from build123d import *

# Parameters (mm, degrees)
CROQUIS1_R              = 2.1
SALIENTE_EXTRUIR1_DEPTH = 4
CROQUIS1_6_R            = 2.1
SALIENTE_EXTRUIR3_DEPTH = 12.65
REDONDEO1_R             = 10


with BuildPart() as part:
    # Croquis1 → Saliente-Extruir1 (new body)
    with BuildSketch(Plane.XY):
        with BuildLine():
            ThreePointArc((10, 54), (0, 64), (-10, 54))
            Line((-10, 54), (-10, -54))
            ThreePointArc((-10, -54), (0, -64), (10, -54))
            Line((10, -54), (10, 54))
        make_face()
        with Locations((0, 54)):
            Circle(CROQUIS1_R, mode=Mode.SUBTRACT)
        with BuildLine():
            Line((6, 38), (6, 22))
            Line((6, 22), (-6, 34))
            Line((-6, 34), (-6, 38))
            ThreePointArc((-6, 38), (0, 44), (6, 38))
        make_face(mode=Mode.SUBTRACT)
        Polygon((6, 16), (6, -16), (-6, -4), (-6, 4), align=None, mode=Mode.SUBTRACT)
        with BuildLine():
            Line((6, -22), (6, -38))
            ThreePointArc((6, -38), (0, -44), (-6, -38))
            Line((-6, -38), (-6, -34))
            Line((-6, -34), (6, -22))
        make_face(mode=Mode.SUBTRACT)
        Polygon((-6, -31), (-6, -7), (6, -19), align=None, mode=Mode.SUBTRACT)
        Polygon((-6, 7), (-6, 31), (6, 19), align=None, mode=Mode.SUBTRACT)
        with Locations((0, -54)):
            Circle(CROQUIS1_R, mode=Mode.SUBTRACT)
    extrude(amount=SALIENTE_EXTRUIR1_DEPTH)

    # Croquis1<6> → Saliente-Extruir3 (add)
    with BuildSketch(Plane.XY):
        with BuildLine():
            Line((10, 47.95), (10, 54))
            ThreePointArc((10, 54), (0, 64), (-10, 54))
            Line((-10, 54), (-10, 47.95))
            Line((-10, 47.95), (10, 47.95))
        make_face()
        with Locations((0, 54)):
            Circle(CROQUIS1_6_R, mode=Mode.SUBTRACT)
    extrude(amount=SALIENTE_EXTRUIR3_DEPTH)

    # Redondeo1
    # the kernel refuses this fillet: 10 mm, written as the material it adds along each edge
    with BuildSketch(Plane(origin=(10, 47.95, 4), x_dir=(0, 0, 1), z_dir=(-1, 0, 0))) as redondeo1_piece_1_section:
        with BuildLine():
            CenterArc((10, -9.908455985), REDONDEO1_R, 97.758619889, 82.241380111)
            Line((0, -9.908455985), (-0.2, -9.908455985))
            Line((-0.2, -9.908455985), (-0.2, 0))
            Line((-0.2, 0), (0, 0.2))
            ThreePointArc((0, 0.2), (4.325, 0.2), (8.623, 0.19816912))
            Line((8.623, 0.19816912), (8.65, 0))
        make_face()
    redondeo1_piece_1 = extrude(amount=20, mode=Mode.PRIVATE)
    redondeo1_piece_1 = redondeo1_piece_1 - Plane(origin=(0, 38, 6.259394391), x_dir=(-1, 0, 0), z_dir=(0, 0, -1)) * Cylinder(6, 80, mode=Mode.PRIVATE)
    add(redondeo1_piece_1)


solid = part.part
Model file for the job. Use its own axes, mm. A direction names the side the tool comes from. Coordinates: 2 decimals unless noted, no trailing zeros. Order: outer loops, then holes, each group sorted by start corner. A loop starts at its lowest first (then second) coordinate and runs counter-clockwise, first axis right, second up. Notation, with made-up numbers: (0, -37) -> (50, -37) arc R20 ccw to (50, -32) -> close; hole circle Ø11 at (50.5, 5.25). An arc over 180 degrees is marked (long way). Return JSON: item names as keys, results as strings. Group by question number.
Item 1: Saw through at D-D on z = 7.75. Write the cut outline in (x, y).
Item 2: Tool access for faces 1 (the flat face through (2, 56, 12.65)), 2 (the flat face through (6, 30, 2)), 3 (the flat face through (2, -24, 4)): list every direction of +Z, -Z, +X, -X, +Y, -Y with a clear straight run to the whole face (end or side of a thin tool).
Item 3: Saw through at C-C on z = 2.5. Write the cut outline in (x, y), then the cut area to 3 significant figures.
Item 4: Pull direction X, two halves, no side cores. Call faces 4 (the flat face through (10, 12.8, 3.6)), 5 (the flat face through (-6, -36, 2)), 6 (the cylindrical face through (0, -64, 2)), 7 (the flat face through (-7, 1, 0)): pulls with the +X half, pulls with the -X half, needs draft (parallel to the pull), parting line crosses it, or undercut.
Item 5: Saw through at B-B on x = 0. State how many separate pieces and enclosed holes the cut face has, then the cut area to 3 significant figures.
Item 6: Flat gauge pins, fed straight in: P1, Ø5, axis at x = -3, z = 9.5, coming from the -Y side; P2, Ø3, axis at x = 1.5, z = 9.5, coming from the -Y side; P3, Ø3.5, axis at x = 0, y = 54, coming from the +Z side; P4, Ø1, axis at x = -2, z = 9, coming from the -Y side. Where does each tip first touch, or does it go through?
Item 7: Wall check: line 1 along X through (y, z) = (28, 2.25); line 2 along Z through (x, y) = (-9, -21); line 3 along Y through (x, z) = (0, 7.5). Give the ranges that are in metal, low to high. Write a range as [from, to].
Item 8: Saw through at A-A on y = 2. Write the cut outline in (x, z).
Values found:
{
 "1": {"outline": "(-10, 45.85) -> (10, 45.85) -> (10, 54) arc R10 ccw to (-10, 54) -> close; hole circle Ø4.2 at (0, 54)"},
 "2": {"face 1": "+Z, +X, -X, +Y, -Y", "face 2": "+Z, -Z", "face 3": "+Z, +X, -X, -Y"},
 "3": {"outline": "(-10, -54) arc R10 ccw to (10, -54) -> (10, 54) arc R10 ccw to (-10, 54) -> close; hole (-6, -38) arc R6 ccw to (6, -38) -> (6, -22) -> (-6, -34) -> close; hole (-6, -31) -> (6, -19) -> (-6, -7) -> close; hole (-6, -4) -> (6, -16) -> (6, 16) -> (-6, 4) -> close; hole (-6, 7) -> (6, 19) -> (-6, 31) -> close; hole (-6, 34) -> (6, 22) -> (6, 38) arc R6 ccw to (-6, 38) -> close; hole circle Ø4.2 at (0, -54); hole circle Ø4.2 at (0, 54)", "area": "1,570 mm2"},
 "4": {"face 4": "pulls with the +X half", "face 5": "undercut", "face 6": "parting line crosses it", "face 7": "needs draft"},
 "5": {"separate pieces": "8", "enclosed holes": "0", "area": "294 mm2"},
 "6": {"P1": "stops at y = 45.18", "P2": "stops at y = 46.04", "P3": "passes through", "P4": "stops at y = 46.39"},
 "7": {"line 1": "x = [-10, -6], [-3, 0], [6, 10]", "line 2": "z = [0, 4]", "line 3": "y = [45.64, 51.9], [56.1, 64]"},
 "8": {"outline": "(-10, 0) -> (-6, 0) -> (-6, 4) -> (-10, 4) -> close; (6, 0) -> (10, 0) -> (10, 4) -> (6, 4) -> close"}
}
